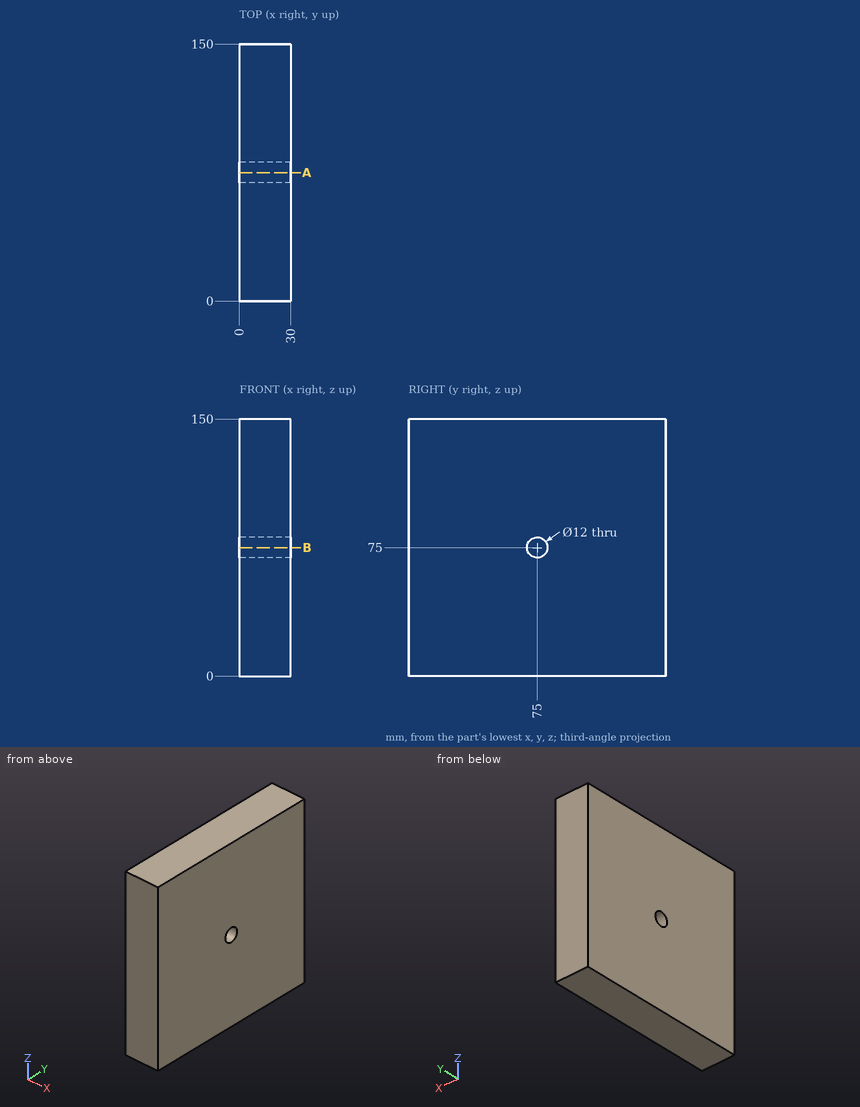
The drawing under review shows one solid part. Ordinate dimensions are in mm from its lowest x, y, z. Give positions to 0.01 mm unless a question says otherwise; leave off trailing zeros. Loops run counter-clockwise (first coordinate to the right, second up) from the corner with the lowest first, then second, coordinate; pieces in that order, holes last. Notation, with made-up numbers: M 13,18 L 43,18 A21 cw 43,55 Z; hole C 14.5,0 d5. An arc over 180 degrees is marked long. One line per question, with ' | ' between items. Start each with the question number.
1. To check wall thickness, follow L1, parallel to Z at x = 14.75, y = 75; L2, parallel to Y at x = 24.75, z = 80; L3, parallel to Y at x = 21, z = 79.5. State the ranges of each line that lie inside material, in increasing order.
2. Insertion check: P1, Ø2, axis at x = 8, y = 23, coming from the -Z side. The pin has a flat end and moves straight along its axis. Give the tip position at first contact, or say it passes through.
3. Add section A-A (y = 75). Write out the cut boundary in (x, z).
Worked out:
1) L1: z = 0 to 69, 81 to 150 | L2: y = 0 to 71.68, 78.32 to 150 | L3: y = 0 to 71.03, 78.97 to 150
2) P1: stops at z = 0
3) outline: M 0,0 L 30,0 L 30,69 L 0,69 Z; M 0,81 L 30,81 L 30,150 L 0,150 Z
